```python
from build123d import *

# Parameters (mm, degrees)
SKETCH_1_R          = 1.35
SKETCH_1_R_2        = 0.85
EXTRUDE_1_DEPTH     = 3
SKETCH_2_R          = 5
SKETCH_2_R_2        = 2.7
EXTRUDE_2_DEPTH     = 3
SKETCH_3_R          = 3
CUT_EXTRUDE_1_DEPTH = 1.5


with BuildPart() as part:
    # Эскиз1 → Бобышка-Вытянуть1 (new body)
    with BuildSketch(Plane.XY):
        with BuildLine():
            Line((6, 16), (6, -2.485281374))
            Line((6, -2.485281374), (2.485281374, -6))
            Line((2.485281374, -6), (-2.485281374, -6))
            Line((-2.485281374, -6), (-6, -2.485281374))
            Line((-6, -2.485281374), (-6, 16))
            ThreePointArc((-6, 16), (0, 22), (6, 16))
        make_face()
        Circle(SKETCH_1_R, mode=Mode.SUBTRACT)
        with Locations((0, 10)):
            Circle(SKETCH_1_R_2, mode=Mode.SUBTRACT)
        with Locations((0, 13)):
            Circle(SKETCH_1_R_2, mode=Mode.SUBTRACT)
        with Locations((0, 16)):
            Circle(SKETCH_1_R_2, mode=Mode.SUBTRACT)
        with Locations((0, 19)):
            Circle(SKETCH_1_R_2, mode=Mode.SUBTRACT)
    extrude(amount=EXTRUDE_1_DEPTH)

    # Эскиз2 → Бобышка-Вытянуть2 (add)
    with BuildSketch(Plane.XY.offset(3)):
        Circle(SKETCH_2_R)
        Circle(SKETCH_2_R_2, mode=Mode.SUBTRACT)
    extrude(amount=EXTRUDE_2_DEPTH)

    # Эскиз3 → Вырез-Вытянуть1 (cut)
    with BuildSketch(Plane(origin=(0, 0, 0), x_dir=(-1, 0, 0), z_dir=(0, 0, -1))):
        Circle(SKETCH_3_R)
    extrude(amount=-CUT_EXTRUDE_1_DEPTH, mode=Mode.SUBTRACT)


solid = part.part
```
For this review, take the finished solid that the model builds, in its own axes (mm). A direction names the side the tool comes from. Coordinates: 2 decimals unless noted, no trailing zeros. Write each loop counter-clockwise with the first axis right and the second up, starting at its lowest first coordinate (ties: lowest second). Pieces come first, ordered by that corner, then holes.
(1) Tool access review of faces 1 (the face through (0, 8, 0)), 2 (the face through (-1.2, -1.2, 3)): name each direction out of +Z, -Z, +X, -X, +Y, -Y from which nothing blocks a thin tool from reaching the whole face with its end or side.
(2) Wall thickness on probe 1 along Y at (x, z) = (0, 2.4); probe 2 along Y at (x, z) = (0, 0.65); probe 3 along X at (y, z) = (0, 2.3): over which ranges is each line inside the solid? List them lowest first.
(3) Add section D-D on z = 4.5. Give the boundary of the cut face in (x, y).
(4) For pin 1 Ø3 at (x, z) = (-1, 5) entering from +Y; pin 2 Ø1 at (x, y) = (0, 13) entering from -Z; pin 3 Ø1.6 at (x, y) = (1.5, -1) entering from +Z; pin 4 Ø4.5 at (x, y) = (0, 0) entering from -Z, all flat-tipped, find the tip position at first contact; note any pin that passes through.
(5) Add section A-A on y = 0. Give the boundary of the cut face in (x, z), then the cut area to 4 significant figures.
(6) Add section B-B on x = -4.75. Give the boundary of the cut face in (y, z), then the cut area to 3 significant figures.
(7) The part is to be moulded in two halves that separate along X. For faces 3 (the face through (-0.18, 18.17, 1.48)), 4 (the face through (0, 22, 1)), 5 (the face through (-4.218, -4.267, 1.479)), say which applies: +X half, -X half, draft (parallel to the pull), parting line (faces both ways), or undercut.
(8) Add section C-C on y = 4.5. Give the boundary of the cut face in (x, z), then the cut area to 3 significant figures.
Answer sheet:
1. face 1: -Z, +X, -X, +Y, -Y
1. face 2: +Z
2. probe 1: y = -6 to -1.35, 1.35 to 9.15, 10.85 to 12.15, 13.85 to 15.15, 16.85 to 18.15, 19.85 to 22
2. probe 2: y = -6 to -3, 3 to 9.15, 10.85 to 12.15, 13.85 to 15.15, 16.85 to 18.15, 19.85 to 22
2. probe 3: x = -6 to -1.35, 1.35 to 6
3. outline: circle Ø10 at (0, 0); hole circle Ø5.4 at (0, 0)
4. pin 1: stops at y = 5
4. pin 2: passes through
4. pin 3: stops at z = 3
4. pin 4: stops at z = 1.5
5. outline: (-6, 0) - (-3, 0) - (-3, 1.5) - (-1.35, 1.5) - (-1.35, 3) - (-2.7, 3) - (-2.7, 6) - (-5, 6) - (-5, 3) - (-6, 3) - close; (1.35, 1.5) - (3, 1.5) - (3, 0) - (6, 0) - (6, 3) - (5, 3) - (5, 6) - (2.7, 6) - (2.7, 3) - (1.35, 3) - close
5. area: 36.75 mm2
6. outline: (-3.74, 0) - (19.67, 0) - (19.67, 3) - (1.56, 3) - (1.56, 6) - (-1.56, 6) - (-1.56, 3) - (-3.74, 3) - close
6. area: 79.6 mm2
7. face 3: undercut
7. face 4: parting line
7. face 5: -X half
8. outline: (-6, 0) - (6, 0) - (6, 3) - (2.18, 3) - (2.18, 6) - (-2.18, 6) - (-2.18, 3) - (-6, 3) - close
8. area: 49.1 mm2
